from build123d import *

# Parameters (mm, degrees)
SKETCH2_W                          = 28
SKETCH2_H                          = 8
BRIDGEBOSS_EXTRUDE2_DEPTH          = 8
GROMMETCUT_EXTRUDE3_DEPTH          = 31.199337741
BRIDGEMOUNTHOLESSKETCH4_R          = 1.55
BRIDGEMOUNTHOLESCUT_EXTRUDE4_DEPTH = 43.532340636
FILLET1_R                          = 3
SKETCH4_R                          = 3
MOUNTHOLESBORECUT_EXTRUDE1_DEPTH   = 4


with BuildPart() as part:
    # Sketch2 → BridgeBoss-Extrude2 (new body)
    with BuildSketch(Plane(origin=(0, 0, 0), x_dir=(1, 0, 0), z_dir=(0, 0, -1))):
        with Locations((14, 27)):
            Rectangle(SKETCH2_W, SKETCH2_H)
    extrude(amount=BRIDGEBOSS_EXTRUDE2_DEPTH)

    # Sketch3 → GrommetCut-Extrude3 (cut, through all)
    with BuildSketch(Plane(origin=(0, -23, 0), x_dir=(1, 0, 0), z_dir=(0, 1, 0))):
        with BuildLine():
            Line((9.75, 8), (18.25, 8))
            ThreePointArc((18.25, 8), (14, 3.75), (9.75, 8))
        make_face()
    extrude(amount=-GROMMETCUT_EXTRUDE3_DEPTH, mode=Mode.SUBTRACT)

    # BridgeMountHolesSketch4 → BridgeMountholesCut-Extrude4 (cut, through all)
    with BuildSketch(Plane(origin=(0, 0, -8), x_dir=(1, 0, 0), z_dir=(0, 0, -1))):
        with Locations(Location((4.875, 27, 0), (0, 0, 270))):
            Circle(BRIDGEMOUNTHOLESSKETCH4_R)
        with Locations(Location((23.125, 27, 0), (0, 0, 270))):
            Circle(BRIDGEMOUNTHOLESSKETCH4_R)
    extrude(amount=-BRIDGEMOUNTHOLESCUT_EXTRUDE4_DEPTH, mode=Mode.SUBTRACT)

    # Fillet1
    fillet1_edges = [part.edges().sort_by_distance(p)[0] for p in [
        (28, -27, 0),
        (0, -27, 0),
    ]]
    fillet(fillet1_edges, radius=FILLET1_R)

    # Sketch4 → MountHolesBoreCut-Extrude1 (cut)
    with BuildSketch(Plane.XY):
        with Locations((4.875, -27)):
            Circle(SKETCH4_R)
        with Locations((23.125, -27)):
            Circle(SKETCH4_R)
    extrude(amount=-MOUNTHOLESBORECUT_EXTRUDE1_DEPTH, mode=Mode.SUBTRACT)


solid = part.part
Can you work these out from the model? Positions are in its coordinate system, mm. A direction names the side the tool comes from. Give positions to 0.01 mm unless a question says otherwise; leave off trailing zeros. Order: outer loops, then holes, each group sorted by start corner. A loop starts at its lowest first (then second) coordinate and runs counter-clockwise, first axis right, second up. Notation, with made-up numbers: M -22.75,73 L 14.25,73 A35 ccw 14.25,111 Z; hole C 13.25,14.5 d11. An arc over 180 degrees is marked long. Use one line per item in the form item = value.
Item 1: If we section it at A-A, the plane z = -7: Write out the boundary of the cut face in (x, y) (3 decimals), and give its area (3 significant figures).
Values follow:
outline = M 0,-31 L 9.869,-31 L 9.869,-23 L 0,-23 Z; M 18.131,-31 L 28,-31 L 28,-23 L 18.131,-23 Z; hole C 4.875,-27 d3.1; hole C 23.125,-27 d3.1
area = 143 mm^2
Item 2: Will this pin go through, and if not, where does the flat tip stop? pin 1 Ø2.5 at (x, y) = (4.875, -27) entering from -Z.
Values follow:
pin_1 = through
Item 3: If we section it at C-C, the plane y = -27: Write out the boundary of the cut face in (x, z) (3 decimals).
Values follow:
outline = M 0,-8 L 3.325,-8 L 3.325,-4 L 1.875,-4 L 1.875,-0.219 A3 ccw 0,-3 Z; M 6.425,-8 L 9.75,-8 A4.25 cw 18.25,-8 L 21.575,-8 L 21.575,-4 L 20.125,-4 L 20.125,0 L 7.875,0 L 7.875,-4 L 6.425,-4 Z; M 24.675,-8 L 28,-8 L 28,-3 A3 ccw 26.125,-0.219 L 26.125,-4 L 24.675,-4 Z
Item 4: If we section it at D-D, the plane z = -3.25: Write out the boundary of the cut face in (x, y) (3 decimals), and give its area (3 significant figures).
Values follow:
outline = M 0,-31 L 28,-31 L 28,-23 L 0,-23 Z; hole C 4.875,-27 d6; hole C 23.125,-27 d6
area = 167 mm^2
Item 5: If I drill on line 1 along X through (y, z) = (-26.5, -2.75); line 2 along X through (y, z) = (-27, -1) (3 decimals); line 3 along Z through (x, y) = (4, -24.5), over which ranges is the centre line in solid material (lowest first)? Write a range as [from, to].
Values follow:
line_1 = [0.01, 1.92], [7.83, 20.17], [26.08, 27.99]
line_2 = [0.764, 1.875], [7.875, 20.125], [26.125, 27.236]
line_3 = [-8, -4]
Item 6: For faces 1 (the flat face through (6.2, -28.3, -4)), 2 (the cylindrical face through (0.86, -27.06, -0.9)), which set-ups out of +Z, -Z, +X, -X, +Y, -Y let a thin tool reach every point of the face, with its end or its side?
Values follow:
face_1 = +Z
face_2 = +Z, -X, +Y, -Y
Item 7: If we section it at B-B, the plane x = 24.25: Write out the boundary of the cut face in (y, z), and give its area (3 significant figures).
Values follow:
outline = M -31,-8 L -28.07,-8 L -28.07,-4 L -29.78,-4 L -29.78,0 L -31,0 Z; M -25.93,-8 L -23,-8 L -23,0 L -24.22,0 L -24.22,-4 L -25.93,-4 Z
area = 33.2 mm^2
Item 8: Thinking about a two-plate mould opening in Y: for faces 3 (the flat face through (14, -31, -3)), 4 (the cylindrical face through (7.736, -26.099, -1.972)), 5 (the flat face through (14, -23, -3)), 6 (the flat face through (23, -25, -8)), which applies, pulls with the +Y half, pulls with the -Y half, needs draft (parallel to the pull), parting line crosses it, or undercut?
Values follow:
face_3 = pulls with the -Y half
face_4 = undercut
face_5 = pulls with the +Y half
face_6 = needs draft
